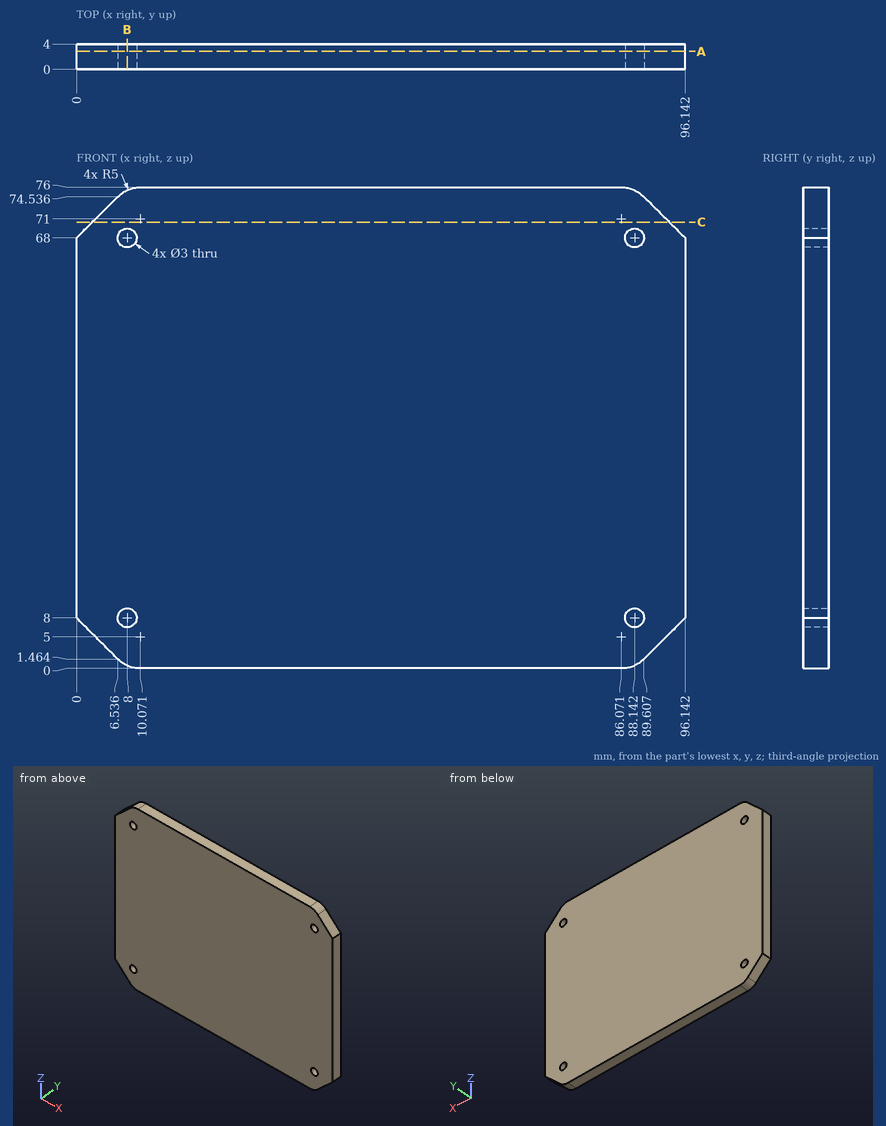
Design review of the part shown in the three views and the two pictorial views. Dimensions are in mm from the part's minimum x, y and z. Round coordinates to 2 decimals unless told otherwise and drop trailing zeros. Order: outer loops, then holes, each group sorted by start corner. A loop starts at its lowest first (then second) coordinate and runs counter-clockwise, first axis right, second up.
(1) For P1, Ø2.5, axis at x = 8, z = 8, coming from the -Y side, flat-tipped, find the tip position at first contact; note if it passes through.
Working result:
P1: passes through
(2) Take a section at C-C, the plane z = 70.5. State the section outline as (x, y) points.
Working result:
outline: (2.5, 0) - (93.64, 0) - (93.64, 4) - (2.5, 4) - close
(3) Wall thickness on L1, parallel to X at y = 2.75, z = 68; L2, parallel to Z at x = 89, y = 0.6; L3, parallel to X at y = 1.5, z = 7 (1 decimal): over which ranges is each line inside the solid? List them lowest first.
Working result:
L1: x = 0 to 6.5, 9.5 to 86.64, 89.64 to 96.14
L2: z = 0.95 to 6.77, 9.23 to 66.77, 69.23 to 75.05
L3: x = 1 to 6.9, 9.1 to 87, 89.3 to 95.1
(4) Take a section at B-B, the plane x = 8. State the section outline as (y, z) points.
Working result:
outline: (0, 0.45) - (4, 0.45) - (4, 6.5) - (0, 6.5) - close; (0, 9.5) - (4, 9.5) - (4, 66.5) - (0, 66.5) - close; (0, 69.5) - (4, 69.5) - (4, 75.55) - (0, 75.55) - close
(5) Take a section at A-A, the plane y = 2.85. State the section outline as (x, z) points (1 decimal), plus the area to 3 significant figures.
Working result:
outline: (0, 8) - (6.5, 1.5) arc R5 ccw to (10.1, 0) - (86.1, 0) arc R5 ccw to (89.6, 1.5) - (96.1, 8) - (96.1, 68) - (89.6, 74.5) arc R5 ccw to (86.1, 76) - (10.1, 76) arc R5 ccw to (6.5, 74.5) - (0, 68) - close; hole circle Ø3 at (8, 8); hole circle Ø3 at (8, 68); hole circle Ø3 at (88.1, 8); hole circle Ø3 at (88.1, 68)
area: 7,150 mm2
